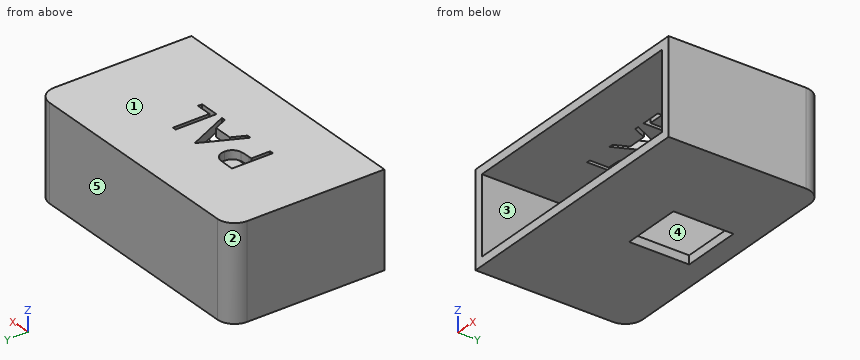
```python
from build123d import *

# Parameters (mm, degrees)
SKETCH1_W           = 30.5
SKETCH1_H           = 18
BOSS_EXTRUDE1_DEPTH = 11
SKETCH3_W           = 28.5
SKETCH3_H           = 9
CUT_EXTRUDE2_DEPTH  = 16
SKETCH4_W           = 7
SKETCH4_H           = 7
CUT_EXTRUDE4_DEPTH  = 5
FILLET4_R           = 2
FILLET5_R           = 2
WRAP2_START         = -1
WRAP2_DEPTH         = 1


# Read off the part's stored shape, not the designer's step: Wrap2
with BuildPart() as part:
    # Sketch1 → Boss-Extrude1 (new body)
    with BuildSketch(Plane.XY):
        with Locations((15.25, 9)):
            Rectangle(SKETCH1_W, SKETCH1_H)
    extrude(amount=BOSS_EXTRUDE1_DEPTH)

    # Sketch3 → Cut-Extrude2 (cut)
    with BuildSketch(Plane(origin=(0, 0, 0), x_dir=(-1, 0, 0), z_dir=(0, -1, 0))):
        with Locations((-15.25, -5.5)):
            Rectangle(SKETCH3_W, SKETCH3_H)
    extrude(amount=-CUT_EXTRUDE2_DEPTH, mode=Mode.SUBTRACT)

    # Sketch4 → Cut-Extrude4 (cut)
    with BuildSketch(Plane(origin=(0, 0, 0), x_dir=(-1, 0, 0), z_dir=(0, 0, -1))):
        with Locations((-16.25, 12)):
            Rectangle(SKETCH4_W, SKETCH4_H)
    extrude(amount=-CUT_EXTRUDE4_DEPTH, mode=Mode.SUBTRACT)

    # Fillet4
    fillet4_edges = [part.edges().sort_by_distance(p)[0] for p in [
        (30.5, 18, 5.5),
    ]]
    fillet(fillet4_edges, radius=FILLET4_R)

    # Fillet5
    fillet5_edges = [part.edges().sort_by_distance(p)[0] for p in [
        (0, 18, 5.5),
    ]]
    fillet(fillet5_edges, radius=FILLET5_R)

    # Wrap2 outline → Wrap2 (cut)
    with BuildSketch(Plane.XY.offset(11).offset(WRAP2_START)):
        with BuildLine():
            add(Edge.make_bspline(
                [(9.556268529, 11.410544446), (9.620509083, 11.41047383), (9.743596838, 11.410338527), (9.920101968, 11.406236319), (10.080407352, 11.400757142), (10.224167335, 11.39316178), (10.35182424, 11.384185705), (10.462800423, 11.371596323), (10.557968176, 11.358451421), (10.61499088, 11.345087293), (10.640996594, 11.338992463)],
                knots=[0, 0, 0, 0, 0.176955752, 0.33905508, 0.486318225, 0.618780923, 0.735618828, 0.838742477, 0.926457068, 1, 1, 1, 1], degree=3))
            Line((9.556268529, 11.410544446), (8.622276642, 11.410544446))
            Line((8.622276642, 11.410544446), (8.622276642, 6.648044446))
            Line((8.622276642, 6.648044446), (9.049680488, 6.648044446))
            Line((9.049680488, 6.648044446), (9.049680488, 8.846121369))
            Line((9.049680488, 8.846121369), (9.390267928, 8.846121369))
            add(Edge.make_bspline(
                [(10.602835536, 8.924351537), (10.572998699, 8.918006552), (10.507609537, 8.904101149), (10.399918904, 8.888577499), (10.274535361, 8.875327406), (10.131630045, 8.865392644), (9.971331228, 8.856887679), (9.793552195, 8.850127522), (9.597943969, 8.846412971), (9.461503455, 8.846221392), (9.390267928, 8.846121369)],
                knots=[0, 0, 0, 0, 0.075173117, 0.164746258, 0.268016881, 0.385911876, 0.517789479, 0.663690977, 0.824413221, 1, 1, 1, 1], degree=3))
            add(Edge.make_bspline(
                [(11.553045872, 10.13310304), (11.552472434, 10.093944708), (11.551350462, 10.017328787), (11.537884445, 9.905242957), (11.519745863, 9.798129719), (11.491855231, 9.696226574), (11.45532594, 9.600138686), (11.412474254, 9.508397653), (11.360789522, 9.422564242), (11.301401379, 9.342326843), (11.23533653, 9.267610141), (11.162874497, 9.198955581), (11.084307817, 9.136765035), (10.999886179, 9.080899081), (10.908786564, 9.032653215), (10.812390633, 8.989440597), (10.709860517, 8.953148904), (10.638909454, 8.934057999), (10.602835536, 8.924351537)],
                knots=[0, 0, 0, 0, 0.070118894, 0.137192353, 0.202016181, 0.264631407, 0.326116547, 0.386010305, 0.445811847, 0.505297697, 0.564633278, 0.624282625, 0.683902032, 0.743952771, 0.805387731, 0.868388031, 0.933084028, 1, 1, 1, 1], degree=3))
            add(Edge.make_bspline(
                [(10.640996594, 11.338992463), (10.673917081, 11.329981881), (10.738982325, 11.312173041), (10.832736958, 11.276503653), (10.921937012, 11.234209707), (11.006888526, 11.186007846), (11.086547574, 11.129829989), (11.162102652, 11.067953387), (11.232886982, 10.998949432), (11.298502519, 10.923592068), (11.358761475, 10.843146353), (11.410645079, 10.756411391), (11.454088913, 10.664847153), (11.491349722, 10.568517329), (11.518167298, 10.466612996), (11.538369686, 10.35984222), (11.551192551, 10.248216445), (11.55242068, 10.171934982), (11.553045872, 10.13310304)],
                knots=[0, 0, 0, 0, 0.062481339, 0.123490383, 0.183411094, 0.243153221, 0.302126735, 0.361709671, 0.421842292, 0.482931901, 0.544552254, 0.60568072, 0.667679738, 0.729984388, 0.794550921, 0.86034562, 0.928907356, 1, 1, 1, 1], degree=3))
        make_face()
        Polygon((19.795834334, 7.136505985), (17.964103565, 7.136505985), (17.964103565, 11.410544446), (17.536699719, 11.410544446), (17.536699719, 6.648044446), (19.795834334, 6.648044446), align=None)
        Polygon((15.513209634, 8.174486754), (16.217281149, 6.648044446), (16.681892026, 6.648044446), (14.483815103, 11.410544446), (14.422757411, 11.410544446), (12.163622795, 6.648044446), (12.630141726, 6.648044446), (13.354247795, 8.174486754), align=None)
    extrude(amount=WRAP2_DEPTH, mode=Mode.SUBTRACT)


solid = part.part
```
Design review of the part built by this model. Coordinates are the model's own, in mm. Face numbers are marked on the shaded views. A direction names the side the tool comes from. Give positions to 0.01 mm unless a question says otherwise; leave off trailing zeros. Order: outer loops, then holes, each group sorted by start corner. A loop starts at its lowest first (then second) coordinate and runs counter-clockwise, first axis right, second up. Notation, with made-up numbers: (39, -27.75) -> (52, -27.75) arc R4 ccw to (52, -22.75) -> close; hole circle Ø6 at (-35.75, -37.75). An arc over 180 degrees is marked (long way). Write each question's results on one line, items separated by ' | '. Start each with the question number.
Q1. Mouldability with a two-part tool opening along X and no side actions: class the marked faces 1, 2 and 3 as +X half, -X half, draft (parallel to the pull), parting line (faces both ways), or undercut.
Q2. Machinability: for the marked faces 4 and 5, which of the approach directions +Z, -Z, +X, -X, +Y, -Y give a long, thin tool a straight path to every point of the face, cutting with its end or side? Answer none if there is none.
Q3. Add section A-A on x = 19. Give the boundary of the cut face in (y, z), and give its area (3 significant figures).
Q4. Wall thickness on L1, parallel to X at y = 14.75, z = 6.75; L2, parallel to Z at x = 27.5, y = 7.5; L3, parallel to Y at x = 3, z = 1.5: over which ranges is each line inside the solid? List them lowest first. Write a range as from..to.
Q5. Add section D-D on z = 1.75. Give the boundary of the cut face in (x, y), and give its area (3 significant figures).
Q6. For pin 1 (4.5 mm diameter, centred on x = 14.5, z = 3.5, fed in from -Y), flat-tipped, find the tip position at first contact; note if it passes through.
Q7. Add section B-B on y = 4.5. Give the boundary of the cut face in (x, z).
Q8. Add section C-C on y = 13.25. Give the boundary of the cut face in (x, z).
Found:
1) face 1: draft | face 2: -X half | face 3: undercut
2) face 4: -Y | face 5: +Z, -Z, +X, -X, +Y
3) outline: (0, 0) -> (8.5, 0) -> (8.5, 1) -> (0, 1) -> close; (0, 10) -> (6.65, 10) -> (6.65, 11) -> (0, 11) -> close; (7.14, 10) -> (16, 10) -> (16, 1) -> (15.5, 1) -> (15.5, 0) -> (18, 0) -> (18, 11) -> (7.14, 11) -> close | area: 46.5 mm2
4) L1: x = 0..1, 29.5..30.5 | L2: z = 0..1, 10..11 | L3: y = 16..18
5) outline: (0, 0) -> (1, 0) -> (1, 16) -> (29.5, 16) -> (29.5, 0) -> (30.5, 0) -> (30.5, 16) arc R2 ccw to (28.5, 18) -> (2, 18) arc R2 ccw to (0, 16) -> close | area: 91.3 mm2
6) pin 1: stops at y = 16
7) outline: (0, 0) -> (30.5, 0) -> (30.5, 11) -> (0, 11) -> close; hole (1, 1) -> (29.5, 1) -> (29.5, 10) -> (1, 10) -> close
8) outline: (0, 0) -> (12.75, 0) -> (12.75, 1) -> (1, 1) -> (1, 10) -> (29.5, 10) -> (29.5, 1) -> (19.75, 1) -> (19.75, 0) -> (30.5, 0) -> (30.5, 11) -> (0, 11) -> close
